Geometry check sheet. Reference: drawing and pictorial views, mm from the part's lowest x, y, z. A direction names the side the tool comes from. Give positions to 0.01 mm unless a question says otherwise; leave off trailing zeros. Write each loop counter-clockwise with the first axis right and the second up, starting at its lowest first coordinate (ties: lowest second). Pieces come first, ordered by that corner, then holes. Notation, with made-up numbers: M 58,43.5 L 108,43.5 A16 ccw 108,71.5 Z; hole C 14.5,43 d8. An arc over 180 degrees is marked long. Write each question's results on one line, items separated by ' | '. Start each with the question number.
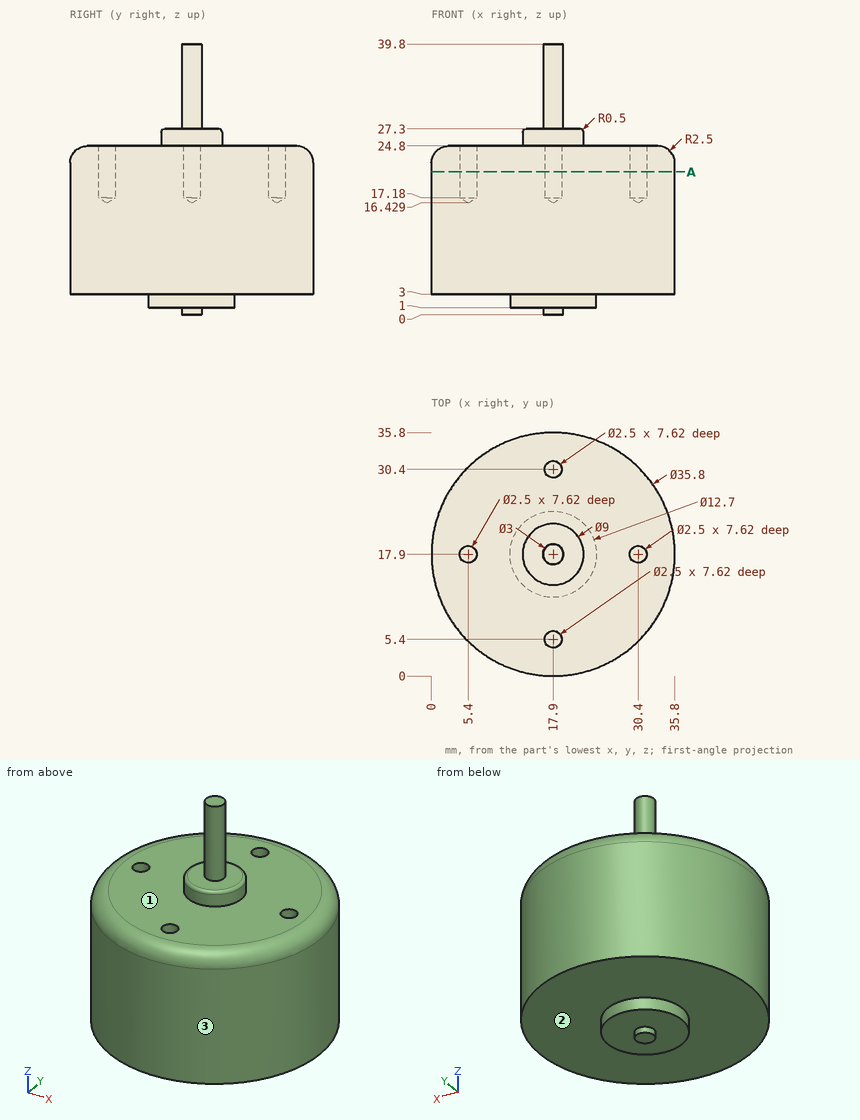
Q1. Depth check by flat-ended pin: pin 1 Ø12 at (x, y) = (10, 22.5) entering from +Z; pin 2 Ø1.5 at (x, y) = (17.9, 5.4) entering from -Z; pin 3 Ø2 at (x, y) = (5.4, 17.9) entering from +Z. Enter the tip coordinate at first touch or a pass-through.
Q2. Tool access check on the marked faces 1, 2 and 3. Record the directions out of +Z, -Z, +X, -X, +Y, -Y that give a thin tool (end or side, any length) a straight path to the whole face; none if there is none.
Q3. Scan lines: L1, parallel to Y at x = 17.9, z = 20.5; L2, parallel to Y at x = 17, z = 17.5; L3, parallel to Y at x = 30, z = 21. Record each from-to range of solid material in increasing order.
Q4. Section check A-A on z = 21. Record the boundary of the cut face in (x, y), plus the area to 3 significant figures.
Check result:
1) pin 1: z = 27.3 | pin 2: z = 3 | pin 3: z = 17.03
2) face 1: +Z | face 2: -Z | face 3: +Z, -Z
3) L1: 0 to 4.15, 6.65 to 29.15, 31.65 to 35.8 | L2: 0.02 to 4.53, 6.27 to 29.53, 31.27 to 35.78 | L3: 4.71 to 16.72, 19.08 to 31.09
4) outline: C 17.9,17.9 d35.8; hole C 5.4,17.9 d2.5; hole C 17.9,5.4 d2.5; hole C 17.9,30.4 d2.5; hole C 30.4,17.9 d2.5 | area: 987 mm^2
